```python
from build123d import *

# Parameters (mm, degrees)
SKETCH1_W           = 42
SKETCH1_H           = 42
SKETCH1_R           = 1.65
BOSS_EXTRUDE1_DEPTH = 1
SKETCH2_R           = 21
BOSS_EXTRUDE2_DEPTH = 20
SKETCH3_R           = 5
BOSS_EXTRUDE3_DEPTH = 10


with BuildPart() as part:
    # Sketch1 → Boss-Extrude1 (new body)
    with BuildSketch(Plane.XY):
        Rectangle(SKETCH1_W, SKETCH1_H)
        with Locations((-17.5, 17.5)):
            Circle(SKETCH1_R, mode=Mode.SUBTRACT)
        with Locations((17.5, 17.5)):
            Circle(SKETCH1_R, mode=Mode.SUBTRACT)
        with Locations((17.5, -17.5)):
            Circle(SKETCH1_R, mode=Mode.SUBTRACT)
        with Locations((-17.5, -17.5)):
            Circle(SKETCH1_R, mode=Mode.SUBTRACT)
    extrude(amount=BOSS_EXTRUDE1_DEPTH)

    # Sketch2 → Boss-Extrude2 (add)
    with BuildSketch(Plane.XY.offset(1)):
        Circle(SKETCH2_R)
    extrude(amount=BOSS_EXTRUDE2_DEPTH)

    # Sketch3 → Boss-Extrude3 (add)
    with BuildSketch(Plane(origin=(0, 0, 0), x_dir=(-1, 0, 0), z_dir=(0, 0, -1))):
        Circle(SKETCH3_R)
    extrude(amount=BOSS_EXTRUDE3_DEPTH)


solid = part.part
```
For this review, take the finished solid that the model builds, in its own axes (mm). A direction names the side the tool comes from. Round coordinates to 2 decimals unless told otherwise and drop trailing zeros. Order: outer loops, then holes, each group sorted by start corner. A loop starts at its lowest first (then second) coordinate and runs counter-clockwise, first axis right, second up. Notation, with made-up numbers: (19, 19) -> (44, 19) arc R33 cw to (44, 53) -> close; hole circle Ø9 at (52, -23.75). An arc over 180 degrees is marked (long way). Use a Markdown table: item, result.
Item 1: Take a section at D-D (z = -7.5). State the section outline as (x, y) points.
Resolved:
| item | result |
|---|---|
| outline | circle Ø10 at (0, 0) |
Item 2: Take a section at B-B (x = 10). State the section outline as (y, z) points.
Resolved:
| item | result |
|---|---|
| outline | (-21, 0) -> (21, 0) -> (21, 1) -> (18.47, 1) -> (18.47, 21) -> (-18.47, 21) -> (-18.47, 1) -> (-21, 1) -> close |
Item 3: Machinability: for faces 1 (the flat face through (-16, 16, 1)), 2 (the cylindrical face through (20.03, 6.31, 10.86)), 3 (the flat face through (16, -16, 1)), which of the approach directions +Z, -Z, +X, -X, +Y, -Y give a long, thin tool a straight path to every point of the face, cutting with its end or side? Answer none if there is none.
Resolved:
| item | result |
|---|---|
| face 1 | +Z, -X, +Y |
| face 2 | +Z |
| face 3 | +Z, +X, -Y |
Item 4: Take a section at C-C (y = -12). State the section outline as (x, z) points, plus the area to 3 significant figures.
Resolved:
| item | result |
|---|---|
| outline | (-21, 0) -> (21, 0) -> (21, 1) -> (17.23, 1) -> (17.23, 21) -> (-17.23, 21) -> (-17.23, 1) -> (-21, 1) -> close |
| area | 731 mm² |
Item 5: For line 1 along Y through (x, z) = (-17.5, 0.65); line 2 along Z through (x, y) = (19, 2.5); line 3 along Y through (x, z) = (0.5, 8.5), list the stretches that pass through material, from the lowest coordinate up. Write a range as [from, to].
Resolved:
| item | result |
|---|---|
| line 1 | y = [-21, -19.15], [-15.85, 15.85], [19.15, 21] |
| line 2 | z = [0, 21] |
| line 3 | y = [-20.99, 20.99] |
Item 6: Take a section at A-A (y = -17.5). State the section outline as (x, z) points, plus the area to 3 significant figures.
Resolved:
| item | result |
|---|---|
| outline | (-21, 0) -> (-19.15, 0) -> (-19.15, 1) -> (-21, 1) -> close; (-15.85, 0) -> (15.85, 0) -> (15.85, 1) -> (11.61, 1) -> (11.61, 21) -> (-11.61, 21) -> (-11.61, 1) -> (-15.85, 1) -> close; (19.15, 0) -> (21, 0) -> (21, 1) -> (19.15, 1) -> close |
| area | 500 mm² |
Item 7: For pin 1 (3 mm diameter, centred on x = 13.5, y = -9.5, fed in from -Z); pin 2 (2.5 mm diameter, centred on x = 17.5, y = -17.5, fed in from +Z); pin 3 (4 mm diameter, centred on x = 17.5, y = 17.5, fed in from +Z); pin 4 (4 mm diameter, centred on x = -5, z = 14.5, fed in from +Y), all flat-tipped, find the tip position at first contact; note any pin that passes through.
Resolved:
| item | result |
|---|---|
| pin 1 | stops at z = 0 |
| pin 2 | passes through |
| pin 3 | stops at z = 1 |
| pin 4 | stops at y = 20.78 |
